Build history of the part. All positions in model axes, mm. Coordinates: 2 decimals unless noted, no trailing zeros. Loops run counter-clockwise (first coordinate to the right, second up) from the corner with the lowest first, then second, coordinate; pieces in that order, holes last.
Item 1: Cut at D-D (x = 80). List the corners of the cut face in (y, z).
Item 2: Mould opens along Z. For faces 1 (the face through (-51.53, 1.52, -0.46)), 2 (the face through (-2, 0, -1)) say: released by +Z, released by -Z, zero draft, split by the parting line, or undercut.
Item 3: Cut at B-B (z = 44). List the corners of the cut face in (x, y), and give its area (3 significant figures).
Item 4: Cut at A-A (z = -65). List the corners of the cut face in (x, y), and give its area (3 significant figures).
Item 5: Drill centre lines: line 1 along X through (y, z) = (1, -65); line 2 along X through (y, z) = (1.1, -50); line 3 along X through (y, z) = (1.05, 16.5). Where is each one in solid material? Low to high.
Item 6: Cut at C-C (y = 2.4). Count the separate pieces of the cut face and the enclosed holes in it, and give its area (3 significant figures).
from build123d import *

# Parameters (mm, degrees)
ESBO_O2_W                = 220
ESBO_O2_H                = 200
RESSALTO_EXTRUS_O1_DEPTH = 3
ESBO_O3_R                = 3.5
ESBO_O3_R_2              = 6
ESBO_O3_R_3              = 8
ESBO_O3_W                = 5
ESBO_O3_H                = 110
ESBO_O3_H_2              = 75
CORTE_EXTRUS_O1_DEPTH    = 149.690954668


with BuildPart() as part:
    # Esboço2 → Ressalto-extrusão1 (new body)
    with BuildSketch(Plane(origin=(0, 0, 0), x_dir=(1, 0, 0), z_dir=(0, 1, 0))):
        Rectangle(ESBO_O2_W, ESBO_O2_H)
    extrude(amount=RESSALTO_EXTRUS_O1_DEPTH)

    # Esboço3 → Corte-extrusão1 (cut, through all)
    with BuildSketch(Plane(origin=(0, 3, 0), x_dir=(1, 0, 0), z_dir=(0, 1, 0))):
        with Locations(Location((-80, 0, 0), (0, 0, 270))):
            Circle(ESBO_O3_R)
        with Locations(Location((-55, 0, 0), (0, 0, 270))):
            Circle(ESBO_O3_R)
        with Locations(Location((-30, 0, 0), (0, 0, 270))):
            Circle(ESBO_O3_R)
        with Locations(Location((-80, -50, 0), (0, 0, 270))):
            Circle(ESBO_O3_R)
        with Locations(Location((-55, -50, 0), (0, 0, 270))):
            Circle(ESBO_O3_R)
        with Locations(Location((-30, -50, 0), (0, 0, 270))):
            Circle(ESBO_O3_R)
        with Locations(Location((-75, 50, 0), (0, 0, 270))):
            Circle(ESBO_O3_R_2)
        with Locations(Location((-35, 50, 0), (0, 0, 270))):
            Circle(ESBO_O3_R_3)
        with Locations(Location((30, 65, 0), (0, 0, 270))):
            Circle(ESBO_O3_R_3)
        with Locations(Location((80, 65, 0), (0, 0, 270))):
            Circle(ESBO_O3_R_3)
        with Locations((70, -20)):
            Rectangle(ESBO_O3_W, ESBO_O3_H)
        with Locations((40, -20)):
            Rectangle(ESBO_O3_W, ESBO_O3_H)
        with Locations((10, -37.5)):
            Rectangle(ESBO_O3_W, ESBO_O3_H_2)
    extrude(amount=-CORTE_EXTRUS_O1_DEPTH, mode=Mode.SUBTRACT)


solid = part.part
Filled sheet:
1. outline: (0, -100) - (3, -100) - (3, -73) - (0, -73) - close; (0, -57) - (3, -57) - (3, 100) - (0, 100) - close
2. face 1: undercut
2. face 2: zero draft
3. outline: (-110, 0) - (7.5, 0) - (7.5, 3) - (-110, 3) - close; (12.5, 0) - (37.5, 0) - (37.5, 3) - (12.5, 3) - close; (42.5, 0) - (67.5, 0) - (67.5, 3) - (42.5, 3) - close; (72.5, 0) - (110, 0) - (110, 3) - (72.5, 3) - close
3. area: 615 mm2
4. outline: (-110, 0) - (22, 0) - (22, 3) - (-110, 3) - close; (38, 0) - (72, 0) - (72, 3) - (38, 3) - close; (88, 0) - (110, 0) - (110, 3) - (88, 3) - close
4. area: 564 mm2
5. line 1: x = -110 to 22, 38 to 72, 88 to 110
5. line 2: x = -110 to -81, -69 to -43, -27 to 110
5. line 3: x = -110 to 7.5, 12.5 to 37.5, 42.5 to 67.5, 72.5 to 110
6. separate pieces: 1
6. enclosed holes: 13
6. area: 41,600 mm2
